Work out the finished part from the listing and answer in its coordinate system (mm). Coordinates: 2 decimals unless noted, no trailing zeros. Loops run counter-clockwise (first coordinate to the right, second up) from the corner with the lowest first, then second, coordinate; pieces in that order, holes last.
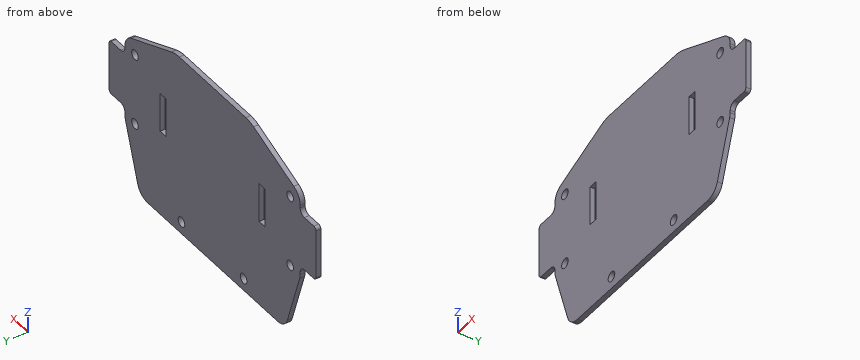
Autodesk Inventor part; units mm, degrees
ref_plane "YZ Plane" through (0, 0, 0) normal (1, 0, 0) x (0, 1, 0)
ref_plane "XZ Plane" through (0, 0, 0) normal (0, 1, 0) x (-1, 0, 0)
ref_plane "XY Plane" through (0, 0, 0) normal (0, 0, 1) x (1, 0, 0)
sketch "Szkic1" plane through (0, 0, 0) normal (0, 1, 0) x (-1, 0, 0)
  arc A0 (49.9, 8) -> (48.9, 9) centre (48.9, 8) ccw
  line L0 (48.9, 9) -> (44.3, 9)
  arc A1 (42.3, 11) -> (44.3, 9) centre (44.3, 11) ccw
  line L1 (42.3, 11) -> (42.3, 11.85)
  arc A2 (42.3, 11.85) -> (39.1714, 16.3842) centre (37.45, 11.85) ccw
  line L2 (39.1714, 16.3842) -> (18, 25)
  line L3 (18, 25) -> (-18, 25)
  line L4 (-18, 25) -> (-39.1714, 16.3842)
  arc A3 (-39.1714, 16.3842) -> (-42.3, 11.85) centre (-37.45, 11.85) ccw
  line L5 (-42.3, 11.85) -> (-42.3, 11)
  arc A4 (-44.3, 9) -> (-42.3, 11) centre (-44.3, 11) ccw
  line L6 (-44.3, 9) -> (-48.9, 9)
  arc A5 (-48.9, 9) -> (-49.9, 8) centre (-48.9, 8) ccw
  line L7 (-49.9, 8) -> (-49.9, -8)
  arc A6 (-49.9, -8) -> (-48.9, -9) centre (-48.9, -8) ccw
  line L8 (-48.9, -9) -> (-44.3, -9)
  arc A7 (-42.3, -11) -> (-44.3, -9) centre (-44.3, -11) ccw
  line L9 (-42.3, -11) -> (-42.3, -11.85)
  arc A8 (-42.3, -11.85) -> (-42.0609, -13.3541) centre (-37.45, -11.85) ccw
  line L10 (-42.0609, -13.3541) -> (-36.1252, -31.5506)
  arc A9 (-36.1252, -31.5506) -> (-31.3717, -35) centre (-31.3717, -30) ccw
  line L11 (-31.3717, -35) -> (31.3717, -35)
  arc A10 (31.3717, -35) -> (36.1252, -31.5506) centre (31.3717, -30) ccw
  line L12 (36.1252, -31.5506) -> (42.0609, -13.3541)
  arc A11 (42.0609, -13.3541) -> (42.3, -11.85) centre (37.45, -11.85) ccw
  line L13 (42.3, -11.85) -> (42.3, -11)
  arc A12 (44.3, -9) -> (42.3, -11) centre (44.3, -11) ccw
  line L14 (44.3, -9) -> (48.9, -9)
  arc A13 (48.9, -9) -> (49.9, -8) centre (48.9, -8) ccw
  line L15 (49.9, -8) -> (49.9, 8)
  line L16 (25.3, -6.4859) -> (22.5, -6.4859)
  line L17 (22.5, -6.4859) -> (22.5, 6.4859)
  line L18 (22.5, 6.4859) -> (25.3, 6.4859)
  line L19 (25.3, 6.4859) -> (25.3, -6.4859)
  circle A14 centre (37.45, 11.85) radius 1.6
  circle A15 centre (37.45, -11.85) radius 1.6
  circle A16 centre (15, -31) radius 1.6
  circle A17 centre (-15, -31) radius 1.6
  circle A18 centre (-37.45, 11.85) radius 1.6
  circle A19 centre (-37.45, -11.85) radius 1.6
  line L20 (-25.3, -6.4859) -> (-25.3, 6.4859)
  line L21 (-25.3, 6.4859) -> (-22.5, 6.4859)
  line L22 (-22.5, 6.4859) -> (-22.5, -6.4859)
  line L23 (-22.5, -6.4859) -> (-25.3, -6.4859)
  point P0 (0, 0)
  point P1 (0, 0)
  point P2 (0, -35)
  point P3 (0, 25)
  dimension "d0" = 36
  dimension "d1" = 60
extrude "Wyciągnięcie proste1" add sketch "Szkic1" along normal blind 1.6
fillet "Zaokrąglenie1" radius 10 2 edges at (-18, 0.8, 25) (18, 0.8, 25)
sketch "Szkic2" plane through (0, 1.6, 0) normal (0, 1, 0) x (1, 0, 0)
  arc A0 (16.0432, -25) -> (19.8125, -24.2624) centre (16.0432, -15) ccw
  line L0 (19.8125, -24.2624) -> (39.1714, -16.3842)
  arc A1 (39.1714, -16.3842) -> (42.3, -11.85) centre (37.45, -11.85) ccw
  line L1 (42.3, -11.85) -> (42.3, -11)
  arc A2 (44.3, -9) -> (42.3, -11) centre (44.3, -11) ccw
  line L2 (44.3, -9) -> (48.9, -9)
  arc A3 (48.9, -9) -> (49.9, -8) centre (48.9, -8) ccw
  line L3 (49.9, -8) -> (49.9, 8)
  arc A4 (49.9, 8) -> (48.9, 9) centre (48.9, 8) ccw
  line L4 (48.9, 9) -> (44.3, 9)
  arc A5 (42.3, 11) -> (44.3, 9) centre (44.3, 11) ccw
  line L5 (42.3, 11) -> (42.3, 11.85)
  arc A6 (42.3, 11.85) -> (42.0609, 13.3541) centre (37.45, 11.85) ccw
  line L6 (42.0609, 13.3541) -> (36.1252, 31.5506)
  arc A7 (36.1252, 31.5506) -> (31.3717, 35) centre (31.3717, 30) ccw
  line L7 (31.3717, 35) -> (-31.3717, 35)
  arc A8 (-31.3717, 35) -> (-36.1252, 31.5506) centre (-31.3717, 30) ccw
  line L8 (-36.1252, 31.5506) -> (-42.0609, 13.3541)
  arc A9 (-42.0609, 13.3541) -> (-42.3, 11.85) centre (-37.45, 11.85) ccw
  line L9 (-42.3, 11.85) -> (-42.3, 11)
  arc A10 (-44.3, 9) -> (-42.3, 11) centre (-44.3, 11) ccw
  line L10 (-44.3, 9) -> (-48.9, 9)
  arc A11 (-48.9, 9) -> (-49.9, 8) centre (-48.9, 8) ccw
  line L11 (-49.9, 8) -> (-49.9, -8)
  arc A12 (-49.9, -8) -> (-48.9, -9) centre (-48.9, -8) ccw
  line L12 (-48.9, -9) -> (-44.3, -9)
  arc A13 (-42.3, -11) -> (-44.3, -9) centre (-44.3, -11) ccw
  line L13 (-42.3, -11) -> (-42.3, -11.85)
  arc A14 (-42.3, -11.85) -> (-39.1714, -16.3842) centre (-37.45, -11.85) ccw
  line L14 (-39.1714, -16.3842) -> (-19.8125, -24.2624)
  arc A15 (-19.8125, -24.2624) -> (-16.0432, -25) centre (-16.0432, -15) ccw
  line L15 (-16.0432, -25) -> (16.0432, -25)
  circle A16 centre (-37.45, -11.85) radius 1.6
  circle A17 centre (37.45, -11.85) radius 1.6
  circle A18 centre (15, 31) radius 1.6
  circle A19 centre (-15, 31) radius 1.6
  circle A20 centre (-37.45, 11.85) radius 1.6
  circle A21 centre (37.45, 11.85) radius 1.6
  line L16 (22.5, -6.4859) -> (22.5, 6.4859)
  line L17 (22.5, 6.4859) -> (25.3, 6.4859)
  line L18 (25.3, 6.4859) -> (25.3, -6.4859)
  line L19 (25.3, -6.4859) -> (22.5, -6.4859)
  line L20 (-22.5, -6.4859) -> (-25.3, -6.4859)
  line L21 (-25.3, -6.4859) -> (-25.3, 6.4859)
  line L22 (-25.3, 6.4859) -> (-22.5, 6.4859)
  line L23 (-22.5, 6.4859) -> (-22.5, -6.4859)
  point P0 (0, 0)
properties part number "plytka_glowna_v3"
1. A cutting plane is placed at A-A, the plane x = 15. Give the vertices of the cut face in (y, z), then the cut area to 3 significant figures.
2. Straight lines are drawn through the part: probe 1 along X at (y, z) = (0.6, -3.5); probe 2 along Z at (x, y) = (15, 1.3); probe 3 along X at (y, z) = (1.25, -30.5). For each, find the intervals that lie inside material, in ascending order.
3. A cutting plane is placed at C-C, the plane x = 37.45. Give the vertices of the cut face in (y, z), then the cut area to 3 significant figures.
4. A cutting plane is placed at D-D, the plane y = 0.75. Count the separate pieces of the cut face and the enclosed holes in it, then the cut area to 3 significant figures.
5. A cutting plane is placed at B-B, the plane z = -2. Give the vertices of the cut face in (x, y), then the cut area to 3 significant figures.
Answers below:
1. outline: (0, -35) - (1.6, -35) - (1.6, -32.6) - (0, -32.6) - close; (0, -29.4) - (1.6, -29.4) - (1.6, 25) - (0, 25) - close
1. area: 90.9 mm2
2. probe 1: x = -49.9 to -25.3, -22.5 to 22.5, 25.3 to 49.9
2. probe 2: z = -35 to -32.6, -29.4 to 25
2. probe 3: x = -36.47 to -16.52, -13.48 to 13.48, 16.52 to 36.47
3. outline: (0, -27.49) - (1.6, -27.49) - (1.6, -13.45) - (0, -13.45) - close; (0, -10.25) - (1.6, -10.25) - (1.6, 10.25) - (0, 10.25) - close; (0, 13.45) - (1.6, 13.45) - (1.6, 17.08) - (0, 17.08) - close
3. area: 61.1 mm2
4. separate pieces: 1
4. enclosed holes: 8
4. area: 4,820 mm2
5. outline: (-49.9, 0) - (-25.3, 0) - (-25.3, 1.6) - (-49.9, 1.6) - close; (-22.5, 0) - (22.5, 0) - (22.5, 1.6) - (-22.5, 1.6) - close; (25.3, 0) - (49.9, 0) - (49.9, 1.6) - (25.3, 1.6) - close
5. area: 151 mm2
